```python
from build123d import *

# Parameters (mm, degrees)
SKETCH1_R           = 16.5
BOSS_EXTRUDE1_DEPTH = 0.5
SKETCH2_R           = 18
BOSS_EXTRUDE2_DEPTH = 3
SKETCH3_R           = 6
CUT_EXTRUDE1_DEPTH  = 26.695330315
SKETCH4_R           = 1.7
CUT_EXTRUDE2_DEPTH  = 26.695330315
CIRPATTERN1_COUNT   = 4
SKETCH5_R           = 1.4
CUT_EXTRUDE3_DEPTH  = 26.695330315
CIRPATTERN2_COUNT   = 4


with BuildPart() as part:
    # Sketch1 → Boss-Extrude1 (new body)
    with BuildSketch(Plane(origin=(0, 0, 0), x_dir=(1, 0, 0), z_dir=(0, 1, 0))):
        with Locations(Location((0, 0, 0), (0, 0, 270))):
            Circle(SKETCH1_R)
    extrude(amount=BOSS_EXTRUDE1_DEPTH)

    # Sketch2 → Boss-Extrude2 (add)
    with BuildSketch(Plane(origin=(0, 0.5, 0), x_dir=(1, 0, 0), z_dir=(0, 1, 0))):
        with Locations(Location((0, 0, 0), (0, 0, 270))):
            Circle(SKETCH2_R)
    extrude(amount=BOSS_EXTRUDE2_DEPTH)

    # Sketch3 → Cut-Extrude1 (cut, through all)
    with BuildSketch(Plane(origin=(0, 0, 0), x_dir=(1, 0, 0), z_dir=(0, 1, 0))):
        with Locations(Location((0, 0, 0), (0, 0, 270))):
            Circle(SKETCH3_R)
    extrude(amount=CUT_EXTRUDE1_DEPTH, mode=Mode.SUBTRACT)

    # Sketch4 → Cut-Extrude2 (cut, through all)
    with BuildSketch(Plane(origin=(0, 0, 0), x_dir=(1, 0, 0), z_dir=(0, 1, 0))):
        with Locations(Location((10.5, 0, 0), (0, 0, 270))):
            Circle(SKETCH4_R)
    cut_extrude2 = extrude(amount=CUT_EXTRUDE2_DEPTH, mode=Mode.SUBTRACT)

    # CirPattern1: Cut-Extrude2 ×4 about axis
    cirpattern1_axis = Axis((0, 0, 0), (0, 1, 0))
    for i in range(1, CIRPATTERN1_COUNT):
        add(cut_extrude2.rotate(cirpattern1_axis, i * 360 / CIRPATTERN1_COUNT), mode=Mode.SUBTRACT)

    # Sketch5 → Cut-Extrude3 (cut, through all)
    with BuildSketch(Plane(origin=(0, 0, 0), x_dir=(1, 0, 0), z_dir=(0, 1, 0))):
        with Locations(Location((9.899494937, 9.899494937, 0), (0, 0, 270))):
            Circle(SKETCH5_R)
    cut_extrude3 = extrude(amount=CUT_EXTRUDE3_DEPTH, mode=Mode.SUBTRACT)

    # CirPattern2: Cut-Extrude3 ×4 about axis
    cirpattern2_axis = Axis((0, 0, 0), (0, 1, 0))
    for i in range(1, CIRPATTERN2_COUNT):
        add(cut_extrude3.rotate(cirpattern2_axis, i * 360 / CIRPATTERN2_COUNT), mode=Mode.SUBTRACT)


solid = part.part
```
The listing builds one solid part. Answer for the finished solid, in the listing's coordinates (mm). A direction names the side the tool comes from. Round coordinates to 2 decimals unless told otherwise and drop trailing zeros. Loops run counter-clockwise (first coordinate to the right, second up) from the corner with the lowest first, then second, coordinate; pieces in that order, holes last.
1) For faces 1 (the face through (10.85, 1.73, -10.93)), 2 (the face through (-15, 0.5, 8)), determine the directions among +Z, -Z, +X, -X, +Y, -Y from which every point of the face is accessible in a straight line to the end or side of a thin tool.
Outcome:
face 1: +Y, -Y
face 2: -Y
2) Given P1, Ø3, axis at x = 0, z = 10.5, coming from the -Y side; P2, Ø2, axis at y = 1.5, z = 0, coming from the +X side; P3, Ø1.5, axis at y = 2, z = -4.5, coming from the -X side; P4, Ø1.5, axis at y = 2.5, z = 13, coming from the +X side, each flat-ended and moving along its own axis, determine where each tip first touches the part or whether it passes through.
Outcome:
P1: passes through
P2: stops at x = 18
P3: stops at x = -17.61
P4: stops at x = 13.19
3) A cutting plane is placed at C-C on y = 2.7. Give the number of separate pieces and of enclosed holes in the cut face, plus the area to 3 significant figures.
Outcome:
separate pieces: 1
enclosed holes: 9
area: 844 mm2
4) A cutting plane is placed at D-D on z = -3.5. Determine the outline of the cut face in (x, y), plus the area to 3 significant figures.
Outcome:
outline: (-17.66, 0.5) - (-16.12, 0.5) - (-16.12, 0) - (-4.87, 0) - (-4.87, 3.5) - (-17.66, 3.5) - close; (4.87, 0) - (16.12, 0) - (16.12, 0.5) - (17.66, 0.5) - (17.66, 3.5) - (4.87, 3.5) - close
area: 87.9 mm2
5) For a pull along Z with two mould halves and no side action, classify faces 3 (the face through (-8, 3.5, 0)), 4 (the face through (10.93, 1.73, 10.85)), 5 (the face through (-10.93, 1.73, -10.85)), 6 (the face through (5.407, 1.979, 17.169)) as released by +Z, released by -Z, zero draft, split by the parting line, or undercut.
Outcome:
face 3: zero draft
face 4: undercut
face 5: undercut
face 6: split by the parting line
6) A cutting plane is placed at A-A on x = 0. Determine the outline of the cut face in (y, z).
Outcome:
outline: (0, -16.5) - (0.5, -16.5) - (0.5, -18) - (3.5, -18) - (3.5, -12.2) - (0, -12.2) - close; (0, -8.8) - (3.5, -8.8) - (3.5, -6) - (0, -6) - close; (0, 6) - (3.5, 6) - (3.5, 8.8) - (0, 8.8) - close; (0, 12.2) - (3.5, 12.2) - (3.5, 18) - (0.5, 18) - (0.5, 16.5) - (0, 16.5) - close
7) Consider line 1 (X direction, y = 2.6, z = 0); line 2 (X direction, y = 0.65, z = -11); line 3 (Z direction, x = -10, y = 1.55). Determine where each line is inside the solid, lowest interval first.
Outcome:
line 1: x = -18 to -12.2, -8.8 to -6, 6 to 8.8, 12.2 to 18
line 2: x = -14.25 to -10.76, -9.03 to -1.62, 1.62 to 9.03, 10.76 to 14.25
line 3: z = -14.97 to -11.3, -8.5 to -1.62, 1.62 to 8.5, 11.3 to 14.97
8) A cutting plane is placed at B-B on z = -10.5. Determine the outline of the cut face in (x, y), plus the area to 3 significant figures.
Outcome:
outline: (-14.62, 0.5) - (-12.73, 0.5) - (-12.73, 0) - (-11.16, 0) - (-11.16, 3.5) - (-14.62, 3.5) - close; (-8.63, 0) - (-1.7, 0) - (-1.7, 3.5) - (-8.63, 3.5) - close; (1.7, 0) - (8.63, 0) - (8.63, 3.5) - (1.7, 3.5) - close; (11.16, 0) - (12.73, 0) - (12.73, 0.5) - (14.62, 0.5) - (14.62, 3.5) - (11.16, 3.5) - close
area: 70.8 mm2
